Part print with two shaded views. Sizes in mm from the minimum x, y, z corner. Coordinates: 2 decimals unless noted, no trailing zeros. Order: outer loops, then holes, each group sorted by start corner. A loop starts at its lowest first (then second) coordinate and runs counter-clockwise, first axis right, second up.
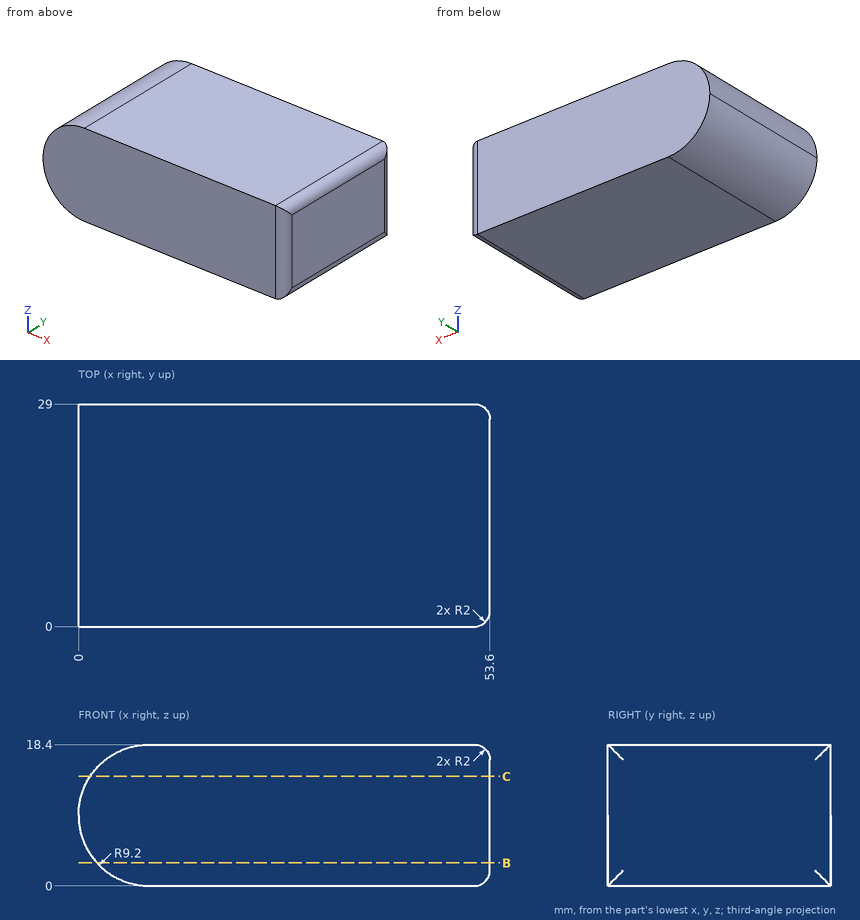
Q1. Cut at B-B on z = 3. Write the cut outline in (x, y), and give its area (3 significant figures).
Results list:
outline: (2.4, 0) - (51.6, 0) arc R2 ccw to (53.6, 2) - (53.6, 27) arc R2 ccw to (51.6, 29) - (2.4, 29) - close
area: 1,480 mm2
Q2. Cut at C-C on z = 14.25. Write the cut outline in (x, y), and give its area (3 significant figures).
Results list:
outline: (1.51, 0) - (51.6, 0) arc R2 ccw to (53.6, 2) - (53.6, 27) arc R2 ccw to (51.6, 29) - (1.51, 29) - close
area: 1,510 mm2
Q3. Wall check: line 1 along X through (y, z) = (22, 12.75); line 2 along X through (y, z) = (15, 5); line 3 along Z through (x, y) = (6.5, 14.25). Give the ranges that are in metal, low to high.
Results list:
line 1: x = 0.71 to 53.6
line 2: x = 1.01 to 53.6
line 3: z = 0.41 to 17.99
